Verification items for the finished model (mm, model axes). A direction names the side the tool comes from. Round coordinates to 2 decimals unless told otherwise and drop trailing zeros. Order: outer loops, then holes, each group sorted by start corner. A loop starts at its lowest first (then second) coordinate and runs counter-clockwise, first axis right, second up. Notation, with made-up numbers: M 76.25,63.5 L 107.25,63.5 A16 cw 107.25,77.5 Z; hole C 57.25,48 d11. An arc over 180 degrees is marked long. Use CSV: the item, a comma, the result in double quotes. Start each with the question number.
Q1. Sectioned sample at B-B (z = 39). Enter the section's corners in (x, y), and give its area (3 significant figures).
Q2. Gauge pin test, flat ends, axial feed: pin 1 Ø15.5 at (x, z) = (76.5, 42.5) entering from -Y; pin 2 Ø5 at (x, z) = (44.5, 102) entering from +Y; pin 3 Ø8 at (x, y) = (63, 132.5) entering from +Z; pin 4 Ø1 at (x, y) = (-10.5, 26) entering from -Z. Record the tip position at first contact, or that the pin passes through.
Q3. Sectioned sample at D-D (x = 26). Enter the section's corners in (y, z), and give its area (3 significant figures).
Q4. Sectioned sample at A-A (x = 69). Enter the section's corners in (y, z), and give its area (3 significant figures).
Q5. Scan lines: line 1 (Z direction, x = 7, y = 22.5); line 2 (Y direction, x = 80.5, z = 29.5); line 3 (Y direction, x = 6.5, z = 59.5). Record each from-to range of solid material in increasing order.
Q6. Set-up check for faces 4 (the face through (84.917, 132, 31)), 5 (the face through (25.305, 20.204, 102.995)), 6 (the face through (33, 76, 0)), 7 (the face through (0, 132, 31)): record each of +Z, -Z, +X, -X, +Y, -Y from which the full face is reachable in a straight line by a thin tool's end or side.
Q7. Mould release check, pull along Y, two halves, no side actions. Record for faces 1 (the face through (42, 145.909, 30)), 2 (the face through (42, 132, 60.637)), 3 (the face through (69, 119.025, 30)): +Y half, -Y half, draft (parallel to the pull), parting line (faces both ways), or undercut.
Q8. Sectioned sample at C-C (y = 48). Enter the section's corners in (x, z), and give its area (3 significant figures).
```python
from build123d import *

# Parameters (mm, degrees)
F0_R     = 57.695631
F1_DEPTH = 65.480502
F2_R     = 41.302375
F3_DEPTH = 141.575145
F4_W     = 26.883833
F4_H     = 60.637102
F5_DEPTH = 84.917324


with BuildPart() as f1:
    # F0 (on Top) → F1 (new body)
    with BuildSketch(Plane.XY):
        with Locations((33.90348, 64.872049)):
            Circle(F0_R)
    extrude(amount=F1_DEPTH)

    # F2 (on Top) → F3 (join)
    with BuildSketch(Plane.XY):
        with Locations((34.258131, 60.523979)):
            Circle(F2_R)
    extrude(amount=F3_DEPTH)

    # F4 (on Right) → F5 (join)
    with BuildSketch(Plane.YZ):
        with Locations((132.467243, 30.318551)):
            Rectangle(F4_W, F4_H)
    extrude(amount=F5_DEPTH)


solid = f1.part
```
Verdict:
1,outline,"M 0,119.03 L 14,119.03 A57.7 ccw long 53.81,119.03 L 84.92,119.03 L 84.92,145.91 L 0,145.91 Z"
1,area,"12,600 mm²"
2,pin 1,"stops at y = 18.89"
2,pin 2,"stops at y = 101.09"
2,pin 3,"stops at z = 60.64"
2,pin 4,"passes through"
3,outline,"M 7.72,0 L 145.91,0 L 145.91,60.64 L 122.02,60.64 L 122.02,65.48 L 100.99,65.48 L 100.99,141.58 L 20.06,141.58 L 20.06,65.48 L 7.72,65.48 Z"
3,area,"15,100 mm²"
4,outline,"M 19.08,0 L 110.67,0 L 110.67,65.48 L 82.86,65.48 L 82.86,141.58 L 38.19,141.58 L 38.19,65.48 L 19.08,65.48 Z; M 119.03,0 L 145.91,0 L 145.91,60.64 L 119.03,60.64 Z"
4,area,"11,000 mm²"
5,line 1,"z = 0 to 65.48"
5,line 2,"y = 30.85 to 98.89, 119.03 to 145.91"
5,line 3,"y = 14.1 to 115.64, 119.03 to 145.91"
6,face 4,"+Z, -Z, +X, +Y"
6,face 5,"+Z"
6,face 6,"-Z, +X, -X, +Y, -Y"
6,face 7,"+Z, -Z, -X, +Y"
7,face 1,"+Y half"
7,face 2,"draft"
7,face 3,"undercut"
8,outline,"M -21.27,0 L 89.08,0 L 89.08,65.48 L 73.62,65.48 L 73.62,141.58 L -5.1,141.58 L -5.1,65.48 L -21.27,65.48 Z"
8,area,"13,200 mm²"
